Here's how the part is built. I have some questions about the finished solid (model axes, mm). Face numbers are marked on the shaded views. A direction names the side the tool comes from. Round coordinates to 2 decimals unless told otherwise and drop trailing zeros. Write each loop counter-clockwise with the first axis right and the second up, starting at its lowest first coordinate (ties: lowest second). Pieces come first, ordered by that corner, then holes. Notation, with made-up numbers: (42, -26) -> (82, -26) arc R20 ccw to (82, 7) -> close; hole circle Ø5 at (-3, -20). An arc over 180 degrees is marked (long way). Put each result on its own line as item: value. Start each with the question number.
1. Which directions (+Z, -Z, +X, -X, +Y, -Y) give clear straight access to the entire face, cutting with the end or side of a thin tool? Please do the marked faces 1 and 2.
2. For pin 1 (5 mm diameter, centred on x = -17.22, y = -0.09, fed in from -Z); pin 2 (8 mm diameter, centred on y = -3, z = 14, fed in from -X); pin 3 (2.5 mm diameter, centred on x = -17.22, y = -22.09, fed in from -Z), each with a flat end and sliding along its axis, tell me the tip position at first contact or that it passes through.
3. Suppose I cut it at C-C (y = -10). Please give me the cut outline in (x, z).
4. Suppose I cut it at D-D (x = -3). Please give me the cut outline in (y, z), then the cut area to 3 significant figures.
5. I need wall thicknesses on probe 1 along X at (y, z) = (-22, 5); probe 2 along Z at (x, y) = (-26.5, -17); probe 3 along X at (y, z) = (-24, 42.5). Which ranges of each line are inside material? Lowest first, please. Write a range as from..to.
6. Suppose I cut it at A-A (z = 38). Please give me the cut outline in (x, y).
7. Suppose I cut it at B-B (y = 1). Please give me the cut outline in (x, z), then the cut area to 3 significant figures.
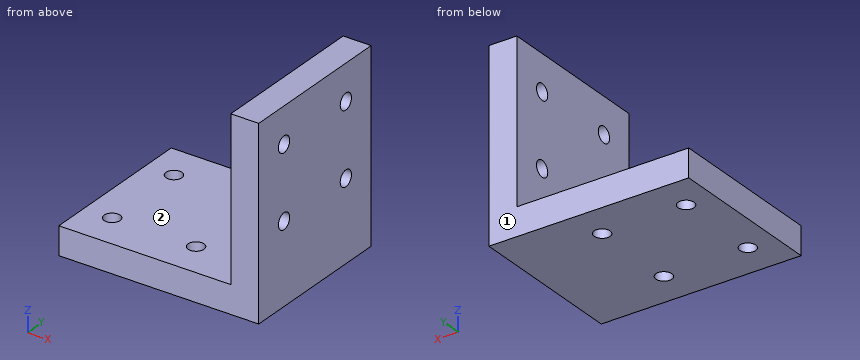
```python
from build123d import *

# Parameters (mm, degrees)
SKETCH1_W           = 50
SKETCH1_H           = 40
BOSS_EXTRUDE1_DEPTH = 7
SKETCH2_W           = 7
SKETCH2_H           = 40
BOSS_EXTRUDE2_DEPTH = 40
SKETCH3_R           = 2
CUT_EXTRUDE1_DEPTH  = 40
SKETCH4_R           = 2
CUT_EXTRUDE2_DEPTH  = 40


with BuildPart() as part:
    # Sketch1 → Boss-Extrude1 (new body)
    with BuildSketch(Plane.XY):
        with Locations((-20.217391304, -11.086956522)):
            Rectangle(SKETCH1_W, SKETCH1_H)
    extrude(amount=BOSS_EXTRUDE1_DEPTH)

    # Sketch2 → Boss-Extrude2 (add)
    with BuildSketch(Plane.XY.offset(7)):
        with Locations((1.282608696, -11.086956522)):
            Rectangle(SKETCH2_W, SKETCH2_H)
    extrude(amount=BOSS_EXTRUDE2_DEPTH)

    # Sketch3 → Cut-Extrude1 (cut)
    with BuildSketch(Plane.XY.offset(7)):
        with Locations((-38.217391304, -0.086956522)):
            Circle(SKETCH3_R)
        with Locations((-38.217391304, -22.086956522)):
            Circle(SKETCH3_R)
        with Locations((-17.217391304, -0.086956522)):
            Circle(SKETCH3_R)
        with Locations((-17.217391304, -22.086956522)):
            Circle(SKETCH3_R)
    extrude(amount=-CUT_EXTRUDE1_DEPTH, mode=Mode.SUBTRACT)

    # Sketch4 → Cut-Extrude2 (cut)
    with BuildSketch(Plane.ZY.offset(2.217391304)):
        with Locations(Location((38, -0.086956522, 0), (0, 0, 270))):
            Circle(SKETCH4_R)
        with Locations(Location((38, -22.086956522, 0), (0, 0, 270))):
            Circle(SKETCH4_R)
        with Locations(Location((20, -0.086956522, 0), (0, 0, 270))):
            Circle(SKETCH4_R)
        with Locations(Location((20, -22.086956522, 0), (0, 0, 270))):
            Circle(SKETCH4_R)
    extrude(amount=-CUT_EXTRUDE2_DEPTH, mode=Mode.SUBTRACT)


solid = part.part
```
Verdict:
1. face 1: +Z, -Z, +X, -X, +Y
1. face 2: +Z, -X, +Y, -Y
2. pin 1: stops at z = 0
2. pin 2: stops at x = -2.22
2. pin 3: passes through
3. outline: (-45.22, 0) -> (4.78, 0) -> (4.78, 47) -> (-2.22, 47) -> (-2.22, 7) -> (-45.22, 7) -> close
4. outline: (-31.09, 0) -> (8.91, 0) -> (8.91, 7) -> (-31.09, 7) -> close
4. area: 280 mm^2
5. probe 1: x = -45.22..-40.22, -36.22..-19.22, -15.22..4.78
5. probe 2: z = 0..7
5. probe 3: x = -2.22..4.78
6. outline: (-2.22, -31.09) -> (4.78, -31.09) -> (4.78, -24.09) -> (-2.22, -24.09) -> close; (-2.22, -20.09) -> (4.78, -20.09) -> (4.78, -2.09) -> (-2.22, -2.09) -> close; (-2.22, 1.91) -> (4.78, 1.91) -> (4.78, 8.91) -> (-2.22, 8.91) -> close
7. outline: (-45.22, 0) -> (-39.9, 0) -> (-39.9, 7) -> (-45.22, 7) -> close; (-36.54, 0) -> (-18.9, 0) -> (-18.9, 7) -> (-36.54, 7) -> close; (-15.54, 0) -> (4.78, 0) -> (4.78, 18.32) -> (-2.22, 18.32) -> (-2.22, 7) -> (-15.54, 7) -> close; (-2.22, 21.68) -> (4.78, 21.68) -> (4.78, 36.32) -> (-2.22, 36.32) -> close; (-2.22, 39.68) -> (4.78, 39.68) -> (4.78, 47) -> (-2.22, 47) -> close
7. area: 536 mm^2
